Can you work these out from the model? Positions are in its coordinate system, mm. Face numbers are marked on the shaded views. A direction names the side the tool comes from. Give positions to 0.01 mm unless a question says otherwise; leave off trailing zeros. Order: outer loops, then holes, each group sorted by start corner. A loop starts at its lowest first (then second) coordinate and runs counter-clockwise, first axis right, second up. Notation, with made-up numbers: (8, -9) -> (55, -9) arc R28 ccw to (55, 19) -> close; hole circle Ø7 at (60, 36). An arc over 180 degrees is marked (long way). Answer as a JSON object with one key per item and string values.
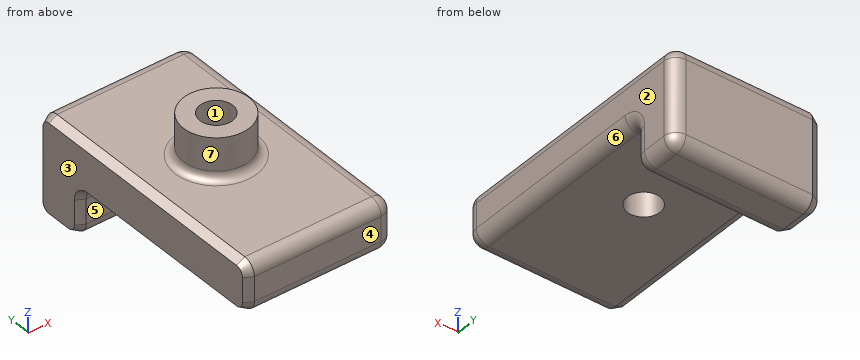
```python
from build123d import *
from OCP.BRepFilletAPI import BRepFilletAPI_MakeChamfer

# Parameters (mm, degrees)
BOSS_EXTRUDE1_DEPTH = 18
SKETCH3_R           = 2
CUT_EXTRUDE1_DEPTH  = 18
FILLET1_R           = 1.5
CHAMFER1_SIZE       = 1
CHAMFER1_SIZE2      = 0.577350269
BOSS_EXTRUDE2_START = 5
SKETCH4_R           = 4
SKETCH4_R_2         = 2
BOSS_EXTRUDE2_DEPTH = 5
FILLET3_R           = 1


with BuildPart() as part:
    # Sketch2 → Boss-Extrude1 (new body)
    with BuildSketch(Plane(origin=(0, 0, 0), x_dir=(0, 0, -1), z_dir=(1, 0, 0))):
        Polygon((0, 0), (0, 32), (12, 32), (12, 26), (6, 26), (6, 0), align=None)
    extrude(amount=BOSS_EXTRUDE1_DEPTH)

    # Sketch3 → Cut-Extrude1 (cut)
    with BuildSketch(Plane.XY):
        with Locations((9, 16)):
            Circle(SKETCH3_R)
    extrude(amount=-CUT_EXTRUDE1_DEPTH, mode=Mode.SUBTRACT)

    # Fillet1
    fillet1_edges = [part.edges().sort_by_distance(p)[0] for p in [
        (9, 0, 0),
        (9, 32, 0),
        (9, 32, -12),
        (9, 26, -12),
        (9, 26, -6),
        (9, 0, -6),
        (18, 26, -9),
        (18, 29, -12),
        (18, 32, -6),
        (18, 16, 0),
        (18, 0, -3),
        (18, 13, -6),
    ]]
    fillet(fillet1_edges, radius=FILLET1_R)

    # Chamfer1: one chamfer whose edges measure the first distance from different faces: ONE call of the kernel's chamfer builder (chamfer() names one face for all edges)
    chamfer1_edges_1 = [part.edges().sort_by_distance(p)[0] for p in [
        (0, 13, -6),
    ]]
    chamfer1_side_1 = [part.faces().sort_by_distance(p)[0] for p in [
        (8.224314761, 12.897259044, -6),
    ]]
    chamfer1_edges_2 = [part.edges().sort_by_distance(p)[0] for p in [
        (0, 16, 0),
    ]]
    chamfer1_side_2 = [part.faces().sort_by_distance(p)[0] for p in [
        (0.333654012, 16, 0),
    ]]
    chamfer1_edges_3 = [part.edges().sort_by_distance(p)[0] for p in [
        (0, 0, -3),
    ]]
    chamfer1_side_3 = [part.faces().sort_by_distance(p)[0] for p in [
        (8.25, 0, -3),
    ]]
    chamfer1_edges_4 = [part.edges().sort_by_distance(p)[0] for p in [
        (0, 32, -6),
    ]]
    chamfer1_side_4 = [part.faces().sort_by_distance(p)[0] for p in [
        (8.25, 32, -6),
    ]]
    chamfer1_edges_5 = [part.edges().sort_by_distance(p)[0] for p in [
        (0, 29, -12),
    ]]
    chamfer1_side_5 = [part.faces().sort_by_distance(p)[0] for p in [
        (8.25, 29, -12),
    ]]
    chamfer1_edges_6 = [part.edges().sort_by_distance(p)[0] for p in [
        (0, 26, -9),
    ]]
    chamfer1_side_6 = [part.faces().sort_by_distance(p)[0] for p in [
        (8.25, 26, -9),
    ]]
    chamfer1_edges_7 = [part.edges().sort_by_distance(p)[0] for p in [
        (0, 31.560660172, -11.560660172),
    ]]
    chamfer1_side_7 = [part.faces().sort_by_distance(p)[0] for p in [
        (8.25, 31.560660172, -11.560660172),
    ]]
    chamfer1_edges_8 = [part.edges().sort_by_distance(p)[0] for p in [
        (0, 26.439339828, -11.560660172),
    ]]
    chamfer1_side_8 = [part.faces().sort_by_distance(p)[0] for p in [
        (8.25, 26.439339828, -11.560660172),
    ]]
    chamfer1_edges_9 = [part.edges().sort_by_distance(p)[0] for p in [
        (0, 0.439339828, -0.439339828),
    ]]
    chamfer1_side_9 = [part.faces().sort_by_distance(p)[0] for p in [
        (8.25, 0.439339828, -0.439339828),
    ]]
    chamfer1_edges_10 = [part.edges().sort_by_distance(p)[0] for p in [
        (0, 0.439339828, -5.560660172),
    ]]
    chamfer1_side_10 = [part.faces().sort_by_distance(p)[0] for p in [
        (8.25, 0.439339828, -5.560660172),
    ]]
    chamfer1_edges_11 = [part.edges().sort_by_distance(p)[0] for p in [
        (0, 31.560660172, -0.439339828),
    ]]
    chamfer1_side_11 = [part.faces().sort_by_distance(p)[0] for p in [
        (8.25, 31.560660172, -0.439339828),
    ]]
    chamfer1_edges_12 = [part.edges().sort_by_distance(p)[0] for p in [
        (0, 25.560660172, -6.439339828),
    ]]
    chamfer1_side_12 = [part.faces().sort_by_distance(p)[0] for p in [
        (8.25, 25.560660172, -6.439339828),
    ]]
    chamfer1 = BRepFilletAPI_MakeChamfer(part.part.solid().wrapped)
    for e in chamfer1_edges_1:
        chamfer1.Add(CHAMFER1_SIZE, CHAMFER1_SIZE2, e.wrapped, chamfer1_side_1[0].wrapped)  # the first distance lies on this face
    for e in chamfer1_edges_2:
        chamfer1.Add(CHAMFER1_SIZE, CHAMFER1_SIZE2, e.wrapped, chamfer1_side_2[0].wrapped)  # the first distance lies on this face
    for e in chamfer1_edges_3:
        chamfer1.Add(CHAMFER1_SIZE, CHAMFER1_SIZE2, e.wrapped, chamfer1_side_3[0].wrapped)  # the first distance lies on this face
    for e in chamfer1_edges_4:
        chamfer1.Add(CHAMFER1_SIZE, CHAMFER1_SIZE2, e.wrapped, chamfer1_side_4[0].wrapped)  # the first distance lies on this face
    for e in chamfer1_edges_5:
        chamfer1.Add(CHAMFER1_SIZE, CHAMFER1_SIZE2, e.wrapped, chamfer1_side_5[0].wrapped)  # the first distance lies on this face
    for e in chamfer1_edges_6:
        chamfer1.Add(CHAMFER1_SIZE, CHAMFER1_SIZE2, e.wrapped, chamfer1_side_6[0].wrapped)  # the first distance lies on this face
    for e in chamfer1_edges_7:
        chamfer1.Add(CHAMFER1_SIZE, CHAMFER1_SIZE2, e.wrapped, chamfer1_side_7[0].wrapped)  # the first distance lies on this face
    for e in chamfer1_edges_8:
        chamfer1.Add(CHAMFER1_SIZE, CHAMFER1_SIZE2, e.wrapped, chamfer1_side_8[0].wrapped)  # the first distance lies on this face
    for e in chamfer1_edges_9:
        chamfer1.Add(CHAMFER1_SIZE, CHAMFER1_SIZE2, e.wrapped, chamfer1_side_9[0].wrapped)  # the first distance lies on this face
    for e in chamfer1_edges_10:
        chamfer1.Add(CHAMFER1_SIZE, CHAMFER1_SIZE2, e.wrapped, chamfer1_side_10[0].wrapped)  # the first distance lies on this face
    for e in chamfer1_edges_11:
        chamfer1.Add(CHAMFER1_SIZE, CHAMFER1_SIZE2, e.wrapped, chamfer1_side_11[0].wrapped)  # the first distance lies on this face
    for e in chamfer1_edges_12:
        chamfer1.Add(CHAMFER1_SIZE, CHAMFER1_SIZE2, e.wrapped, chamfer1_side_12[0].wrapped)  # the first distance lies on this face
    add(Compound.cast(chamfer1.Shape()), mode=Mode.REPLACE)

    # Sketch4 → Boss-Extrude2 (add)
    with BuildSketch(Plane.XY.offset(BOSS_EXTRUDE2_START)):
        with Locations(Location((9, 16, 0), (0, 0, 180))):
            Circle(SKETCH4_R)
        with Locations((9, 16)):
            Circle(SKETCH4_R_2, mode=Mode.SUBTRACT)
    extrude(amount=-BOSS_EXTRUDE2_DEPTH)

    # Fillet3
    fillet3_edges = [part.edges().sort_by_distance(p)[0] for p in [
        (13, 16, 0),
    ]]
    fillet(fillet3_edges, radius=FILLET3_R)


solid = part.part
```
1. If we mould it in two halves opening along X, with no side actions, what happens to the marked faces 1, 2, 3 and 4? For each: +X half, -X half, draft (parallel to the pull), parting line (faces both ways), or undercut.
Worked answers:
{"face 1": "undercut", "face 2": "+X half", "face 3": "-X half", "face 4": "draft"}
2. For the marked faces 5, 6 and 7, which set-ups out of +Z, -Z, +X, -X, +Y, -Y let a thin tool reach every point of the face, with its end or its side?
Worked answers:
{"face 5": "-Z, +X, -X, -Y", "face 6": "-Z, +X, -Y", "face 7": "+Z"}
3. Will these pins go through, and if not, where does the flat tip stop? pin 1 Ø5 at (x, z) = (11, -9.5) entering from -Y; pin 2 Ø2.5 at (x, y) = (9, 16) entering from +Z; pin 3 Ø6 at (x, y) = (15.5, 22.5) entering from -Z; pin 4 Ø2.5 at (x, z) = (7, -9) entering from -Y.
Worked answers:
{"pin 1": "y = 25.91", "pin 2": "through", "pin 3": "z = -6.38", "pin 4": "y = 26"}
4. Please list where these lines run through material, in increasing order: L1, parallel to Y at x = 9, z = 2; L2, parallel to Z at x = 12.5, y = 3; L3, parallel to Y at x = 1, z = -9.5.
Worked answers:
{"L1": "12 to 14, 18 to 20", "L2": "-6 to 0", "L3": "26 to 32"}
5. If we section it at D-D on z = -8.5: Please give me the cut outline in (x, y).
Worked answers:
{"outline": "(0, 26.58) -> (1, 26) -> (16.5, 26) arc R1.5 ccw to (18, 27.5) -> (18, 30.5) arc R1.5 ccw to (16.5, 32) -> (1, 32) -> (0, 31.42) -> close"}
6. If we section it at C-C on z = -2.5: Please give me the cut outline in (x, y).
Worked answers:
{"outline": "(0, 0.58) -> (1, 0) -> (16.5, 0) arc R1.5 ccw to (18, 1.5) -> (18, 30.5) arc R1.5 ccw to (16.5, 32) -> (1, 32) -> (0, 31.42) -> close; hole circle Ø4 at (9, 16)"}
7. If we section it at A-A on y = 16: Please give me the cut outline in (x, z), then the cut area to 3 significant figures.
Worked answers:
{"outline": "(0, -5.42) -> (1, -6) -> (7, -6) -> (7, 5) -> (5, 5) -> (5, 1) arc R1 cw to (4, 0) -> (1, 0) -> (0, -0.58) -> close; (11, -6) -> (16.5, -6) arc R1.5 ccw to (18, -4.5) -> (18, -1.5) arc R1.5 ccw to (16.5, 0) -> (14, 0) arc R1 cw to (13, 1) -> (13, 5) -> (11, 5) -> close", "area": "103 mm²"}
8. If we section it at B-B on x = 9: Please give me the cut outline in (y, z), then the cut area to 3 significant figures.
Worked answers:
{"outline": "(0, -4.5) arc R1.5 ccw to (1.5, -6) -> (14, -6) -> (14, 5) -> (12, 5) -> (12, 1) arc R1 cw to (11, 0) -> (1.5, 0) arc R1.5 ccw to (0, -1.5) -> close; (18, -6) -> (24.5, -6) arc R1.5 cw to (26, -7.5) -> (26, -10.5) arc R1.5 ccw to (27.5, -12) -> (30.5, -12) arc R1.5 ccw to (32, -10.5) -> (32, -1.5) arc R1.5 ccw to (30.5, 0) -> (21, 0) arc R1 cw to (20, 1) -> (20, 5) -> (18, 5) -> close", "area": "222 mm²"}
